Read the model definition and answer for the solid it produces. Units are mm, in the model's axes. Round coordinates to 2 decimals unless told otherwise and drop trailing zeros. Loops run counter-clockwise (first coordinate to the right, second up) from the corner with the lowest first, then second, coordinate; pieces in that order, holes last. Notation, with made-up numbers: M 88.25,24 L 138.25,24 A16 ccw 138.25,53 Z; hole C 78.25,64 d4. An arc over 180 degrees is marked long. Write each question's results on one line, items separated by ' | '.
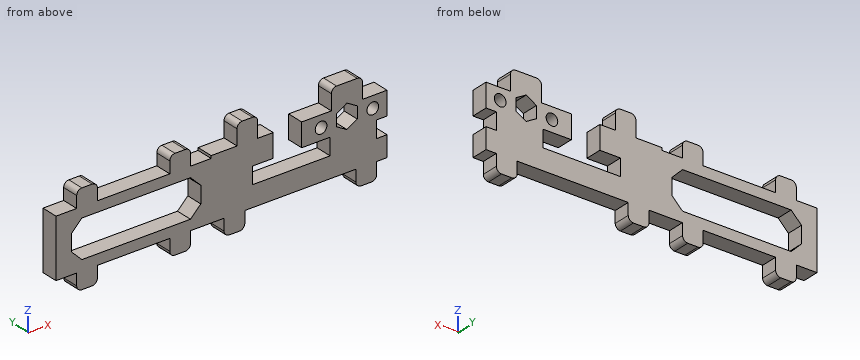
Autodesk Inventor part; units mm, degrees
ref_plane "YZ Plane" through (0, 0, 0) normal (1, 0, 0) x (0, 1, 0)
ref_plane "XZ Plane" through (0, 0, 0) normal (0, 1, 0) x (-1, 0, 0)
ref_plane "XY Plane" through (0, 0, 0) normal (0, 0, 1) x (1, 0, 0)
sketch "Sketch1" plane through (0, 0, 0) normal (0, 1, 0) x (-1, 0, 0)
  line L0 (0, 0) -> (128, 0)
  line L1 (128, 0) -> (128, 22.5)
  line L2 (52, 14.5) -> (52, 8)
  line L3 (52, 8) -> (22, 8)
  line L4 (22, 8) -> (22, 14.5)
  circle A0 centre (5.5, 19) radius 2.25
  circle A1 centre (5.5, 19) radius 4.5 construction
  circle A2 centre (25.5, 19) radius 2.25
  circle A3 centre (25.5, 19) radius 4.5 construction
  line L5 (33, 14.5) -> (44, 14.5) construction
  circle A4 centre (38.5, 19.599) radius 7.5 construction
  circle A5 centre (38.5, 19.599) radius 4 construction
  line L6 (33, 23.5) -> (33, 14.5)
  line L7 (44, 14.5) -> (44, 23.5)
  line L8 (22, 14.5) -> (33, 14.5)
  line L9 (44, 14.5) -> (52, 14.5)
  line L10 (0, 14.5) -> (4, 14.5)
  line L11 (4, 14.5) -> (4, 8)
  line L12 (4, 8) -> (0, 8)
  line L13 (0, 23.5) -> (0, 14.5)
  line L14 (0, 8) -> (0, 0)
  line L15 (9.5, 23.5) -> (9.5, 29.5)
  line L16 (11.5, 31.5) -> (19.5, 31.5)
  line L17 (21.5, 29.5) -> (21.5, 23.5)
  arc A6 (11.5, 31.5) -> (9.5, 29.5) centre (11.5, 29.5) ccw
  arc A7 (21.5, 29.5) -> (19.5, 31.5) centre (19.5, 29.5) ccw
  line L18 (33, 23.5) -> (21.5, 23.5)
  line L19 (9.5, 23.5) -> (0, 23.5)
  line L20 (50, 23.5) -> (50, 29.5)
  line L21 (52, 31.5) -> (56, 31.5)
  line L22 (58, 29.5) -> (58, 23.5)
  arc A8 (52, 31.5) -> (50, 29.5) centre (52, 29.5) ccw
  arc A9 (58, 29.5) -> (56, 31.5) centre (56, 29.5) ccw
  line L23 (68, 23.5) -> (58, 23.5)
  line L24 (50, 23.5) -> (44, 23.5)
  line L25 (68, 23.5) -> (68, 22.5)
  line L26 (68, 22.5) -> (128, 22.5)
  line L27 (19.5, 17.2896) -> (15.5, 14.9802)
  line L28 (15.5, 14.9802) -> (11.5, 17.2896)
  line L29 (11.5, 17.2896) -> (11.5, 21.9084)
  line L30 (11.5, 21.9084) -> (15.5, 24.2178)
  line L31 (15.5, 24.2178) -> (19.5, 21.9084)
  line L32 (19.5, 21.9084) -> (19.5, 17.2896)
  point P0 (15.5, 19.599)
  point P1 (0, 19)
  point P2 (15.5, 31.5)
  point P3 (15.5, 19.599)
  dimension "d0" = 6.5
  dimension "d1" = 8
  dimension "d3" = 4.5
  dimension "d4" = 9
  dimension "d5" = 4.5
  dimension "d6" = 9
  dimension "d8" = 11
  dimension "d9" = 8
  dimension "d10" = 15
  dimension "d11" = 9
  dimension "d12" = 4
  dimension "d13" = 5.5
  dimension "d14" = 10
  dimension "d15" = 10
  dimension "d16" = 2
  dimension "d17" = 12
  dimension "d18" = 8
  dimension "d19" = 23
  dimension "d20" = 30
  dimension "d21" = 18
  dimension "d23" = 2
  dimension "d24" = 8
  dimension "d25" = 6
  dimension "d26" = 8
  dimension "d27" = 10
  dimension "d29" = 60
  dimension "d30" = 8
extrude "Extrusion1" add sketch "Sketch1" along normal blind 6.5
sketch "Sketch2" plane through (0, 6.5, 0) normal (0, 1, 0) x (1, 0, 0)
  line L0 (-128, 0) -> (-128, -22.5)
  line L1 (-128, -22.5) -> (-68, -22.5)
  line L2 (-68, -22.5) -> (-68, -23.5)
  line L3 (-120, -22.5) -> (-112, -22.5)
  line L4 (-112, -22.5) -> (-112, -27)
  line L5 (-114, -29) -> (-118, -29)
  line L6 (-120, -27) -> (-120, -22.5)
  line L7 (-84, -22.5) -> (-76, -22.5)
  line L8 (-76, -22.5) -> (-76, -27)
  line L9 (-78, -29) -> (-82, -29)
  line L10 (-84, -27) -> (-84, -22.5)
  arc A0 (-84, -27) -> (-82, -29) centre (-82, -27) ccw
  arc A1 (-78, -29) -> (-76, -27) centre (-78, -27) ccw
  arc A2 (-114, -29) -> (-112, -27) centre (-114, -27) ccw
  arc A3 (-120, -27) -> (-118, -29) centre (-118, -27) ccw
  dimension "d33" = 2
  dimension "d34" = 8
  dimension "d35" = 6.5
  dimension "d36" = 8
  dimension "d37" = 8
  dimension "d38" = 8
extrude "Extrusion2" add sketch "Sketch2" against normal blind 6.5
sketch "Sketch3" plane through (0, 6.5, 0) normal (0, 1, 0) x (1, 0, 0)
  line L0 (0, 0) -> (-128, 0)
  line L1 (-112, -27) -> (-112, -22.5)
  line L2 (-76, -27) -> (-76, -22.5)
  line L3 (0, -8) -> (0, 0)
  line L4 (-120, 0) -> (-112, 0)
  line L5 (-112, 0) -> (-112, 4.5)
  line L6 (-114, 6.5) -> (-118, 6.5)
  line L7 (-120, 4.5) -> (-120, 0)
  line L8 (-84, 0) -> (-76, 0)
  line L9 (-76, 0) -> (-76, 4.5)
  line L10 (-78, 6.5) -> (-82, 6.5)
  line L11 (-84, 4.5) -> (-84, 0)
  line L12 (-63, 0) -> (-55, 0)
  line L13 (-55, 0) -> (-55, 4.5)
  line L14 (-57, 6.5) -> (-61, 6.5)
  line L15 (-63, 4.5) -> (-63, 0)
  line L16 (-12, 0) -> (-4, 0)
  line L17 (-4, 0) -> (-4, 4.5)
  line L18 (-6, 6.5) -> (-10, 6.5)
  line L19 (-12, 4.5) -> (-12, 0)
  arc A0 (-118, 6.5) -> (-120, 4.5) centre (-118, 4.5) ccw
  arc A1 (-112, 4.5) -> (-114, 6.5) centre (-114, 4.5) ccw
  arc A2 (-82, 6.5) -> (-84, 4.5) centre (-82, 4.5) ccw
  arc A3 (-76, 4.5) -> (-78, 6.5) centre (-78, 4.5) ccw
  arc A4 (-61, 6.5) -> (-63, 4.5) centre (-61, 4.5) ccw
  arc A5 (-55, 4.5) -> (-57, 6.5) centre (-57, 4.5) ccw
  arc A6 (-10, 6.5) -> (-12, 4.5) centre (-10, 4.5) ccw
  arc A7 (-4, 4.5) -> (-6, 6.5) centre (-6, 4.5) ccw
  dimension "d41" = 2
  dimension "d42" = 6.5
  dimension "d43" = 8
  dimension "d44" = 8
  dimension "d45" = 8
  dimension "d46" = 8
  dimension "d47" = 4
  dimension "d48" = 43
extrude "Extrusion3" add sketch "Sketch3" against normal blind 6.5
sketch "Sketch4" plane through (0, 0, 0) normal (0, -1, 0) x (1, 0, 0)
  line L0 (-112, 22.5) -> (-84, 22.5)
  line L1 (-128, 0) -> (-128, 22.5)
  line L2 (-84, 0) -> (-112, 0)
  line L3 (-63, 0) -> (-76, 0)
  line L4 (-4, -4.5) -> (-4, 0)
  line L5 (-122, 14.5) -> (-122, 8)
  line L6 (-122, 8) -> (-118, 4)
  line L7 (-118, 4) -> (-76, 4)
  line L8 (-76, 4) -> (-72, 8)
  line L9 (-72, 8) -> (-72, 14.5)
  line L10 (-72, 14.5) -> (-76, 18.5)
  line L11 (-76, 18.5) -> (-118, 18.5)
  line L12 (-118, 18.5) -> (-122, 14.5)
  line L13 (-68, 22.5) -> (-68, 0) construction
  dimension "d52" = 45
  dimension "d53" = 4
  dimension "d54" = 4
  dimension "d55" = 6
  dimension "d56" = 4
  dimension "d57" = 4
extrude "Extrusion4" cut sketch "Sketch4" against normal blind 6.5
properties part number "x_iddler_wall_upper"
Item 1: The part is cut by section C-C (z = 13). Determine the outline of the cut face in (x, y).
Outcome:
outline: M -128,0 L -122,0 L -122,6.5 L -128,6.5 Z; M -72,0 L -52,0 L -52,6.5 L -72,6.5 Z; M -22,0 L -4,0 L -4,6.5 L -22,6.5 Z
Item 2: Flat-ended cylindrical pins translate along their axes: pin 1 (2 mm diameter, centred on y = 3, z = -2.5, fed in from -X); pin 2 (3 mm diameter, centred on x = -1, y = 5, fed in from -Z); pin 3 (2 mm diameter, centred on x = -122, y = 2.5, fed in from +Z). Find the tip coordinate at first contact, or state that the pin passes through.
Outcome:
pin 1: stops at x = -120 | pin 2: stops at z = 0 | pin 3: stops at z = 22.5
Item 3: Straight lines are drawn through the part: line 1 (Z direction, x = -25.5, y = 3.25); line 2 (X direction, y = 1.5, z = -3.5); line 3 (Z direction, x = -86.5, y = 3). For each, find the intervals that lie inside material, in ascending order.
Outcome:
line 1: z = 0 to 8, 14.5 to 16.75, 21.25 to 23.5 | line 2: x = -120 to -112, -84 to -76, -63 to -55, -12 to -4 | line 3: z = 0 to 4, 18.5 to 22.5
Item 4: The part is cut by section A-A (x = -92). Determine the outline of the cut face in (y, z).
Outcome:
outline: M 0,0 L 6.5,0 L 6.5,4 L 0,4 Z; M 0,18.5 L 6.5,18.5 L 6.5,22.5 L 0,22.5 Z
Item 5: The part is cut by section B-B (z = -2). Determine the outline of the cut face in (x, y), plus the area to 3 significant figures.
Outcome:
outline: M -120,0 L -112,0 L -112,6.5 L -120,6.5 Z; M -84,0 L -76,0 L -76,6.5 L -84,6.5 Z; M -63,0 L -55,0 L -55,6.5 L -63,6.5 Z; M -12,0 L -4,0 L -4,6.5 L -12,6.5 Z | area: 208 mm2
Item 6: The part is cut by section D-D (x = -25.5). Determine the outline of the cut face in (y, z).
Outcome:
outline: M 0,0 L 6.5,0 L 6.5,8 L 0,8 Z; M 0,14.5 L 6.5,14.5 L 6.5,16.75 L 0,16.75 Z; M 0,21.25 L 6.5,21.25 L 6.5,23.5 L 0,23.5 Z
